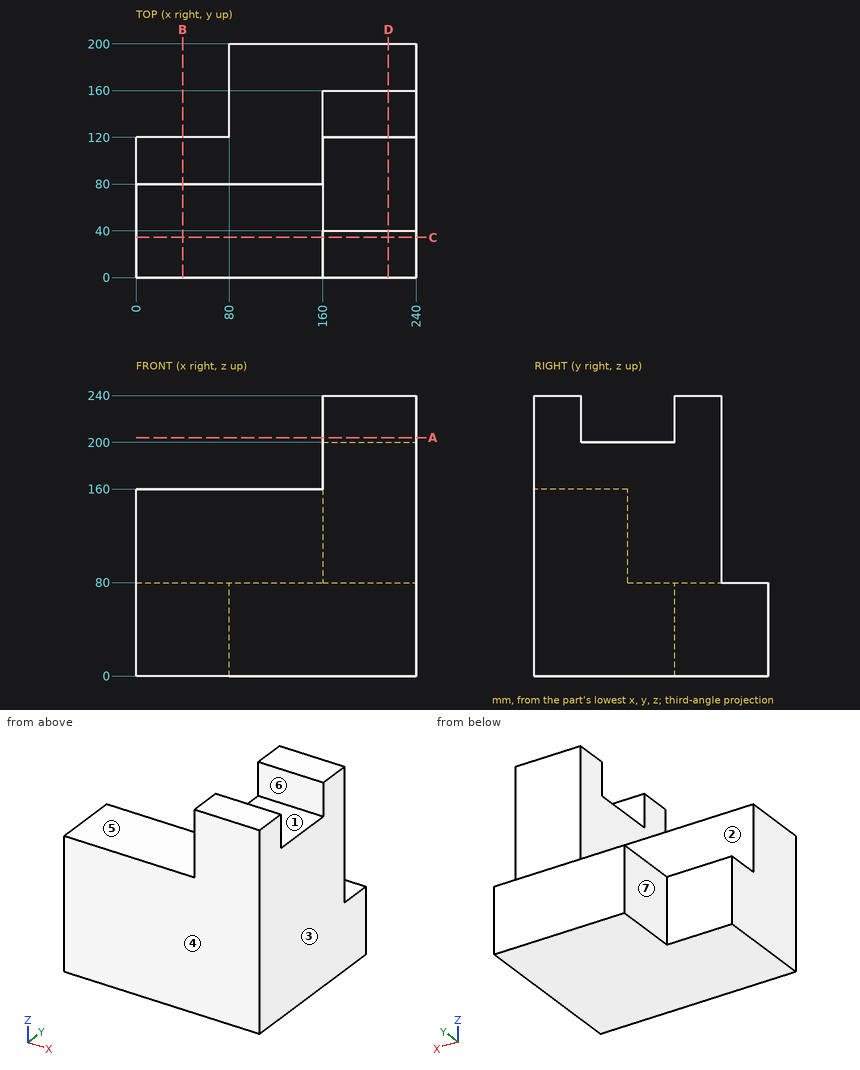
Part print with two shaded views. Sizes in mm from the minimum x, y, z corner. A direction names the side the tool comes from. Give positions to 0.01 mm unless a question says otherwise; leave off trailing zeros. Order: outer loops, then holes, each group sorted by start corner. A loop starts at its lowest first (then second) coordinate and runs counter-clockwise, first axis right, second up.
(1) Mould opens along Y. For the marked faces 1, 2, 3 and 4 say: released by +Y, released by -Y, zero draft, split by the parting line, or undercut.
(2) Drill centre lines: L1, parallel to X at y = 190.5, z = 40; L2, parallel to Y at x = 166, z = 194.5; L3, parallel to Z at x = 88, y = 134. Where is each one in solid material? Low to high.
(3) Tool access for the marked faces 5, 6 and 7: list every direction of +Z, -Z, +X, -X, +Y, -Y with a clear straight run to the whole face (end or side of a thin tool).
(4) Saw through at A-A, the plane z = 204. Give the cut face in (x, y), then the cut area to 3 significant figures.
(5) Saw through at B-B, the plane x = 40. Give the cut face in (y, z), then the cut area to 3 significant figures.
(6) Saw through at C-C, the plane y = 34.5. Give the cut face in (x, z), then the cut area to 3 significant figures.
(7) Saw through at D-D, the plane x = 216. Give the cut face in (y, z).
(8) Flat gauge pins, fed straight in: pin 1 (12 mm diameter, centred on y = 64.5, z = 174.5, fed in from -X); pin 2 (10 mm diameter, centred on x = 187.5, z = 159.5, fed in from -Y); pin 3 (24 mm diameter, centred on y = 169, z = 31, fed in from -X); pin 4 (10 mm diameter, centred on y = 167, z = 118.5, fed in from -X). Where does each tip first touch, or does it go through?
Results found:
1. face 1: undercut
1. face 2: released by +Y
1. face 3: zero draft
1. face 4: released by -Y
2. L1: x = 80 to 240
2. L2: y = 0 to 160
2. L3: z = 0 to 80
3. face 5: +Z, -X, +Y, -Y
3. face 6: +Z, +X, -X
3. face 7: +Z, -Z, -X, +Y
4. outline: (160, 0) - (240, 0) - (240, 40) - (160, 40) - close; (160, 120) - (240, 120) - (240, 160) - (160, 160) - close
4. area: 6,400 mm2
5. outline: (0, 0) - (120, 0) - (120, 80) - (80, 80) - (80, 160) - (0, 160) - close
5. area: 16,000 mm2
6. outline: (0, 0) - (240, 0) - (240, 240) - (160, 240) - (160, 160) - (0, 160) - close
6. area: 44,800 mm2
7. outline: (0, 0) - (200, 0) - (200, 80) - (160, 80) - (160, 240) - (120, 240) - (120, 200) - (40, 200) - (40, 240) - (0, 240) - close
8. pin 1: stops at x = 160
8. pin 2: stops at y = 0
8. pin 3: stops at x = 80
8. pin 4: passes through
